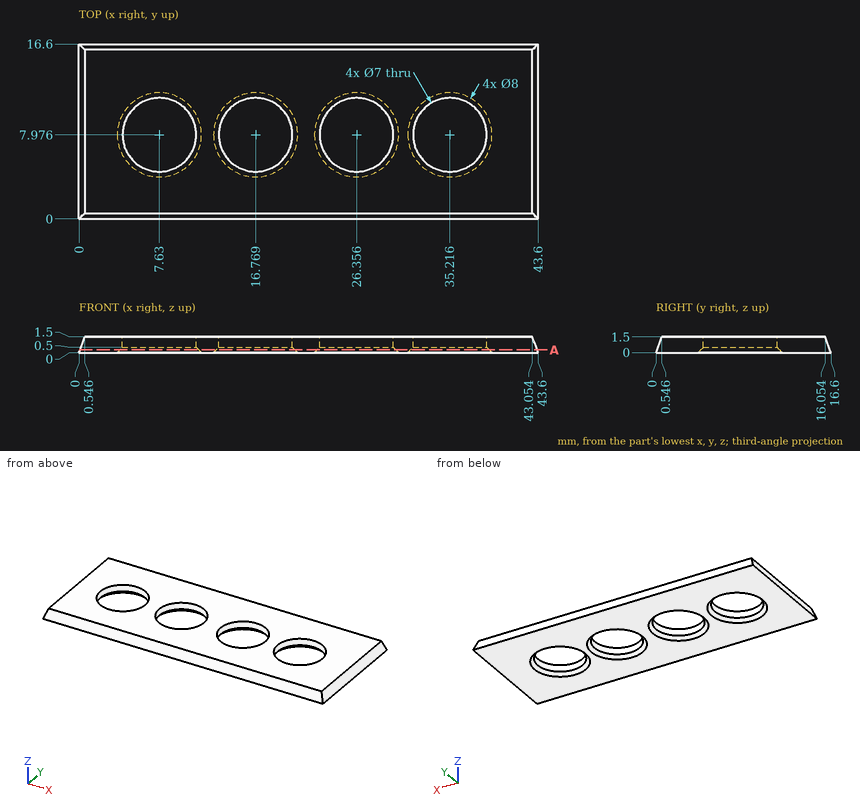
Check sheet for the drawn part. Datum: minimum x, y, z corner. Units: mm. Coordinates: 2 decimals unless noted, no trailing zeros. Answer as CSV lines item,"result".
1) Cross-section at A-A, the plane z = 0.25. Count the separate pieces of the cut face and the enclosed holes in it, then the cut area to 3 significant figures.
Found:
separate pieces,"1"
enclosed holes,"4"
area,"536 mm2"
2) Depth check by flat-ended pin: pin 1 (9 mm diameter, centred on x = 16.77, y = 7.98, fed in from -Z); pin 2 (1 mm diameter, centred on x = 6, y = 11, fed in from -Z) (1 decimal). Enter the tip coordinate at first touch or a pass-through.
Found:
pin 1,"stops at z = 0"
pin 2,"stops at z = 0.1"
3) Thickness scan on L1, parallel to X at y = 8.5, z = 0.6 (1 decimal); L2, parallel to X at y = 5, z = 1 (1 decimal); L3, parallel to Y at x = 25.5, z = 0.8. Record the ranges inside material, lowest first. Write a range as from..to.
Found:
L1,"x = 0.2..4.2, 11.1..13.3, 20.2..22.9, 29.8..31.8, 38.7..43.4"
L2,"x = 0.4..5.8, 9.5..14.9, 18.6..24.5, 28.2..33.4, 37.1..43.2"
L3,"y = 0.29..4.58, 11.37..16.31"
